Here's how the part is built. I have some questions about the finished solid (model axes, mm). A direction names the side the tool comes from. Give positions to 0.01 mm unless a question says otherwise; leave off trailing zeros. Write each loop counter-clockwise with the first axis right and the second up, starting at its lowest first coordinate (ties: lowest second). Pieces come first, ordered by that corner, then holes. Notation, with made-up numbers: (9, 2.25) -> (51, 2.25) arc R9 ccw to (51, 10.25) -> close; hole circle Ø10 at (55, 25.25). An arc over 180 degrees is marked (long way). Use one line per item in the form item = value.
```python
from build123d import *

# Parameters (mm, degrees)
EXTRUDE_1_DEPTH     = 50
SKETCH_2_W          = 10
SKETCH_2_H          = 10
CUT_EXTRUDE_1_DEPTH = 10


with BuildPart() as part:
    # 草圖1 → 填料-伸長1 (new body)
    with BuildSketch(Plane.XY):
        with BuildLine():
            Line((-74.049587352, 0), (0, 0))
            Line((0, 0), (0, 26.398160535))
            Line((0, 26.398160535), (53.133849001, 49.556160033))
            Line((53.133849001, 49.556160033), (15.64046603, -30.209174327))
            Line((15.64046603, -30.209174327), (53.133849001, -19.181708747))
            Line((53.133849001, -19.181708747), (15.64046603, -105.195940269))
            Line((15.64046603, -105.195940269), (0, -105.195940269))
            add(Edge.make_bspline(
                [(-74.049587352, 0), (11.284113354, -28.926204628), (0, -105.195940269)],
                knots=[0, 0, 0, 1, 1, 1], degree=2))
        make_face()
    extrude(amount=EXTRUDE_1_DEPTH)

    # 草圖2 → 除料-伸長1 (cut)
    with BuildSketch(Plane.ZY):
        with Locations((25, 5)):
            Rectangle(SKETCH_2_W, SKETCH_2_H)
    extrude(amount=-CUT_EXTRUDE_1_DEPTH, mode=Mode.SUBTRACT)


solid = part.part
```
Q1. I want a section at B-B, the plane y = 15. Write out the boundary of the cut face in (x, z), and give its area (3 significant figures).
Result set:
outline = (0, 0) -> (36.89, 0) -> (36.89, 50) -> (0, 50) -> close
area = 1,840 mm2
Q2. I want a section at C-C, the plane x = 18.5. Write out the boundary of the cut face in (y, z).
Result set:
outline = (-98.64, 0) -> (-29.37, 0) -> (-29.37, 50) -> (-98.64, 50) -> close; (-24.13, 0) -> (34.46, 0) -> (34.46, 50) -> (-24.13, 50) -> close
Q3. If I drill on line 1 along Y through (x, z) = (34, 2.5); line 2 along Y through (x, z) = (23, 37); line 3 along X through (y, z) = (-48, 12.5), over which ranges is the centre line in solid material (lowest first)? Write a range as from..to.
Result set:
line_1 = -63.08..-24.81, 8.85..41.22
line_2 = -88.31..-28.04, -14.55..36.42
line_3 = -8.36..40.57
Q4. If we mould it in two halves opening along Y, with no side actions, what happens to faces 5 (the face through (13, -27, 0)), 6 (the face through (34.65, -61.59, 24.65)), 7 (the face through (10, 5, 25))? For each: +Y half, -Y half, draft (parallel to the pull), parting line (faces both ways), or undercut.
Result set:
face_5 = draft
face_6 = -Y half
face_7 = undercut
Q5. Which directions (+Z, -Z, +X, -X, +Y, -Y) give clear straight access to the entire face, cutting with the end or side of a thin tool? Please do faces 1 (the face through (0, 13, 25)), 2 (the face through (8, -105.196, 25)), 3 (the face through (34.125, -24.773, 24.65)), 4 (the face through (5, 5, 20)).
Result set:
face_1 = +Z, -Z, -X, +Y
face_2 = +Z, -Z, +X, -X, -Y
face_3 = +Z, -Z
face_4 = -X
Q6. I want a section at A-A, the plane x = 44.5. Write out the boundary of the cut face in (y, z), and give its area (3 significant figures).
Result set:
outline = (-38.99, 0) -> (-21.72, 0) -> (-21.72, 50) -> (-38.99, 50) -> close; (31.19, 0) -> (45.79, 0) -> (45.79, 50) -> (31.19, 50) -> close
area = 1,590 mm2
Q7. Will these pins go through, and if not, where does the flat tip stop? pin 1 Ø4 at (y, z) = (-44, 34) entering from +X; pin 2 Ø12 at (x, z) = (-41.5, 38.5) entering from +Y; pin 3 Ø2 at (y, z) = (-71, 30.5) entering from +X.
Result set:
pin_1 = 43.19
pin_2 = 0
pin_3 = 30.98
